The listing builds one solid part. Answer for the finished solid, in the listing's coordinates (mm). Face numbers are marked on the shaded views. A direction names the side the tool comes from. Give positions to 0.01 mm unless a question says otherwise; leave off trailing zeros. Write each loop counter-clockwise with the first axis right and the second up, starting at its lowest first coordinate (ties: lowest second). Pieces come first, ordered by that corner, then holes. Notation, with made-up numbers: (23, -6.5) - (33, -6.5) arc R26 cw to (33, 12.5) - close; hole circle Ø6 at (48, 18). An arc over 180 degrees is marked (long way). Answer as CSV lines item,"result". Start each with the question number.
(1) Find section B-B (z = -5.5). Write down the section's boundary in (x, y) (3 decimals).
(2) Find section A-A (z = 6.5). Write down the section's boundary in (x, y) (3 decimals).
(3) Each of these flat-tipped pins is pushed along its axis until it touches: pin 1 Ø21 at (y, z) = (-2.5, 11.5) entering from -X; pin 2 Ø19 at (x, y) = (-5.5, -6) entering from +Z. Where does it stop, or does it pass through?
(4) For a pull along X with two mould halves and no side action, classify the marked faces 1, 2 and 3 as pulls with the +X half, pulls with the -X half, needs draft (parallel to the pull), parting line crosses it, or undercut.
(5) Straight lines are drawn through the part: probe 1 along X at (y, z) = (-4, 7.5) (3 decimals); probe 2 along X at (y, z) = (-3.5, -4) (3 decimals); probe 3 along X at (y, z) = (-2, 15.5). For each, find the intervals that lie inside material, in ascending order.
(6) Find section C-C (y = -11.5). Write down the section's boundary in (x, z) (3 decimals), then the cut area to 3 significant figures.
(7) For the marked faces 4, 5 and 6, determine the directions among +Z, -Z, +X, -X, +Y, -Y from which every point of the face is accessible in a straight line to the end or side of a thin tool.
(8) Find section D-D (y = 7). Write down the section's boundary in (x, z), then the cut area to 3 significant figures.
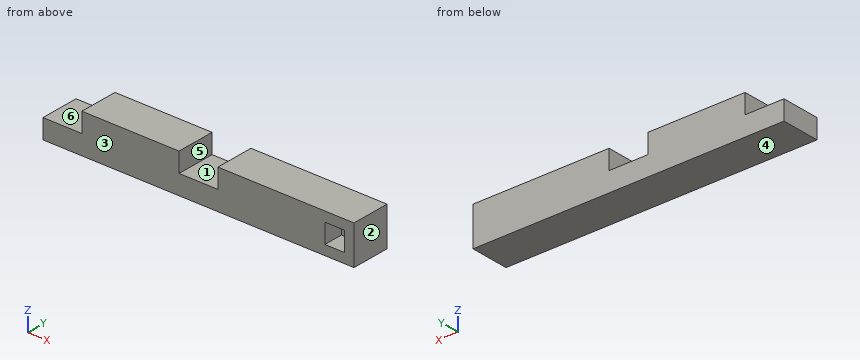
from build123d import *

# Parameters (mm, degrees)
F0_W     = 304.8
F0_H     = 38.1
F1_DEPTH = 19.05
F2_W     = 38.1
F2_H     = 38.1
F3_DEPTH = 19.05
F4_W     = 19.05
F4_H     = 19.05
F5_DEPTH = 19.05
F6_W     = 38.1
F6_H     = 38.1
F7_DEPTH = 19.05


with BuildPart() as f1:
    # F0 (on Top) → F1 (new body, symmetric)
    with BuildSketch(Plane.XY):
        Rectangle(F0_W, F0_H)
    extrude(amount=F1_DEPTH, both=True)

    # F2 (on Top) → F3 (cut)
    with BuildSketch(Plane.XY):
        Rectangle(F2_W, F2_H)
    extrude(amount=F3_DEPTH, mode=Mode.SUBTRACT)

    # F4 (on face) → F5 (cut)
    with BuildSketch(Plane.XZ.offset(19.05)):
        with Locations((133.35, 0)):
            Rectangle(F4_W, F4_H)
    extrude(amount=-F5_DEPTH, mode=Mode.SUBTRACT)

    # F6 (on face) → F7 (cut)
    with BuildSketch(Plane.XY.offset(19.05)):
        with Locations((-133.35, 0)):
            Rectangle(F6_W, F6_H)
    extrude(amount=-F7_DEPTH, mode=Mode.SUBTRACT)


solid = f1.part
Result set:
1,outline,"(-152.4, -19.05) - (123.825, -19.05) - (123.825, 0) - (142.875, 0) - (142.875, -19.05) - (152.4, -19.05) - (152.4, 19.05) - (-152.4, 19.05) - close"
2,outline,"(-114.3, -19.05) - (-19.05, -19.05) - (-19.05, 19.05) - (-114.3, 19.05) - close; (19.05, -19.05) - (123.825, -19.05) - (123.825, 0) - (142.875, 0) - (142.875, -19.05) - (152.4, -19.05) - (152.4, 19.05) - (19.05, 19.05) - close"
3,pin 1,"x = -114.3"
3,pin 2,"z = 0"
4,face 1,"undercut"
4,face 2,"pulls with the +X half"
4,face 3,"needs draft"
5,probe 1,"-114.3 to -19.05, 19.05 to 123.825, 142.875 to 152.4"
5,probe 2,"-152.4 to 123.825, 142.875 to 152.4"
5,probe 3,"-114.3 to -19.05, 19.05 to 152.4"
6,outline,"(-152.4, -19.05) - (152.4, -19.05) - (152.4, 19.05) - (19.05, 19.05) - (19.05, 0) - (-19.05, 0) - (-19.05, 19.05) - (-114.3, 19.05) - (-114.3, 0) - (-152.4, 0) - close; hole (123.825, -9.525) - (142.875, -9.525) - (142.875, 9.525) - (123.825, 9.525) - close"
6,area,"9,800 mm^2"
7,face 4,"-Z, +X, -X, +Y, -Y"
7,face 5,"+Z, +Y, -Y"
7,face 6,"+Z, -X, +Y, -Y"
8,outline,"(-152.4, -19.05) - (152.4, -19.05) - (152.4, 19.05) - (19.05, 19.05) - (19.05, 0) - (-19.05, 0) - (-19.05, 19.05) - (-114.3, 19.05) - (-114.3, 0) - (-152.4, 0) - close"
8,area,"10,200 mm^2"
